Geometry check sheet. Reference: drawing and pictorial views, mm from the part's lowest x, y, z. A direction names the side the tool comes from. Round coordinates to 2 decimals unless told otherwise and drop trailing zeros. Loops run counter-clockwise (first coordinate to the right, second up) from the corner with the lowest first, then second, coordinate; pieces in that order, holes last. Notation, with made-up numbers: M 14,79.25 L 48,79.25 A11 cw 48,99.25 Z; hole C -27.5,-16 d11. An arc over 180 degrees is marked long. One line per question, with ' | ' between items. Start each with the question number.
(1) Thickness scan on probe 1 along Y at (x, z) = (29, 47.5); probe 2 along X at (y, z) = (45.5, 27); probe 3 along Z at (x, y) = (24, 18.5) (1 decimal). Record the ranges inside material, lowest first. Write a range as [from, to].
(2) Section check D-D (y = 6). Record the boundary of the cut face in (x, z), and give its area (3 significant figures).
(3) Go/stop test with flat-tipped pins: P1, Ø6, axis at x = 40.64, z = 12.53, coming from the -Y side; P2, Ø4.5, axis at x = 25, z = 45, coming from the +Y side; P3, Ø4, axis at x = 7, z = 41.5, coming from the +Y side; P4, Ø8, axis at y = 27, z = 33.5, coming from the +X side. Record where each tip stops, or that it passes through.
(4) Section check B-B (y = 24.5). Count the separate pieces of the cut face and the enclosed holes in it, and give its area (3 significant figures).
(5) Draft check along Z on the marked faces 3, 4 and 5. Enter one of: +Z half, -Z half, draft (parallel to the pull), parting line (faces both ways), or undercut.
(6) Section check C-C (x = 45). Record the boundary of the cut face in (y, z).
(7) Section check A-A (x = 25). Record the boundary of the cut face in (y, z), and give its area (3 significant figures).
(8) Tool access check on the marked faces 1 and 2. Record the directions out of +Z, -Z, +X, -X, +Y, -Y that give a thin tool (end or side, any length) a straight path to the whole face; none if there is none.
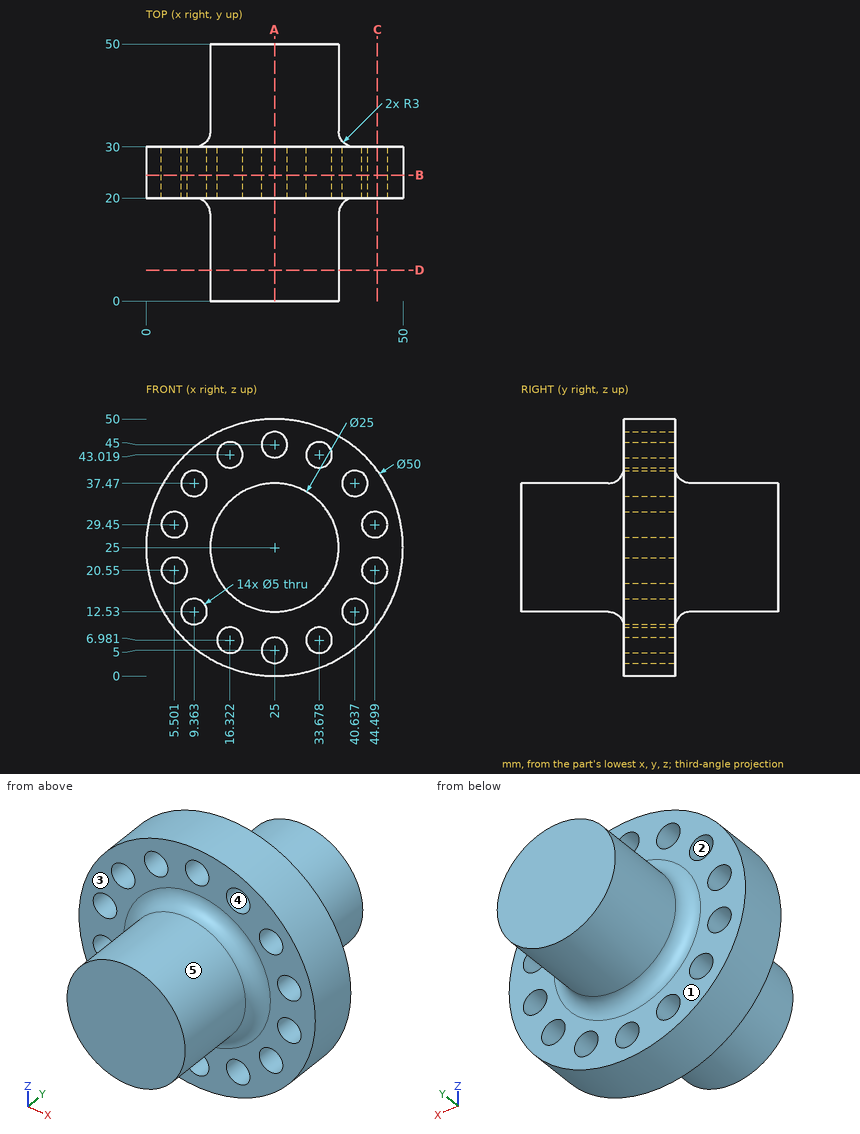
The answers:
1) probe 1: [20, 30] | probe 2: [12.66, 37.34] | probe 3: [12.1, 37.9]
2) outline: C 25,25 d25 | area: 491 mm²
3) P1: y = 20 | P2: through | P3: y = 30 | P4: x = 49.59
4) separate pieces: 1 | enclosed holes: 14 | area: 1,690 mm²
5) face 3: draft | face 4: undercut | face 5: parting line
6) outline: M 20,10 L 30,10 L 30,18.1 L 20,18.1 Z; M 20,23 L 30,23 L 30,27 L 20,27 Z; M 20,31.9 L 30,31.9 L 30,40 L 20,40 Z
7) outline: M 0,12.5 L 17,12.5 A3 cw 20,9.5 L 20,7.5 L 30,7.5 L 30,9.5 A3 cw 33,12.5 L 50,12.5 L 50,37.5 L 33,37.5 A3 cw 30,40.5 L 30,42.5 L 20,42.5 L 20,40.5 A3 cw 17,37.5 L 0,37.5 Z; M 20,0 L 30,0 L 30,2.5 L 20,2.5 Z; M 20,47.5 L 30,47.5 L 30,50 L 20,50 Z | area: 1,410 mm²
8) face 1: +Y | face 2: +Y, -Y
